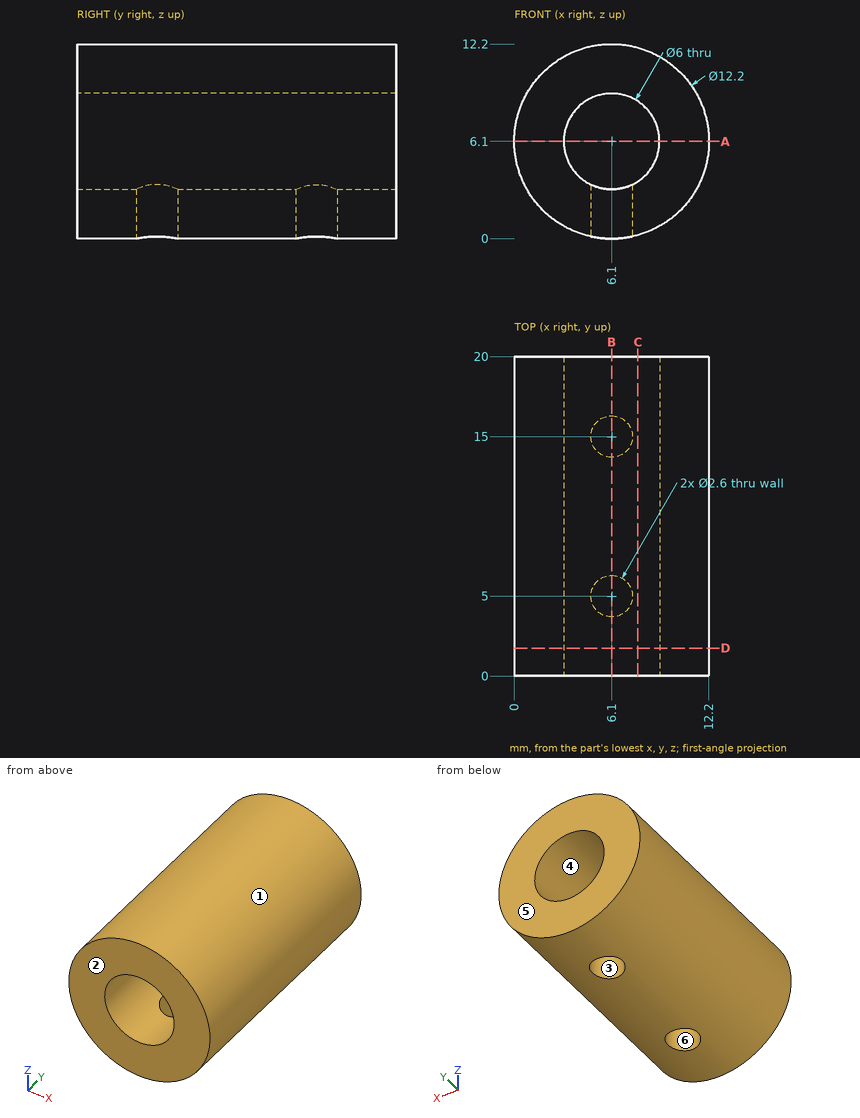
The drawing under review shows one solid part. Ordinate dimensions are in mm from its lowest x, y, z. A direction names the side the tool comes from. Coordinates: 2 decimals unless noted, no trailing zeros. Order: outer loops, then holes, each group sorted by start corner. A loop starts at its lowest first (then second) coordinate and runs counter-clockwise, first axis right, second up. Notation, with made-up numbers: (7.25, 47) -> (50.25, 47) arc R11 ccw to (50.25, 64) -> close; hole circle Ø11 at (67, 48.5). An arc over 180 degrees is marked (long way). Use CSV: the item, a comma, the result in double quotes. Start each with the question number.
Item 1: We need section C-C, the plane x = 7.75. Give the boundary of the cut face in (y, z), then the cut area to 3 significant figures.
Item 2: Insertion check: pin 1 (5 mm diameter, centred on x = 5.5, y = 3, fed in from -Z); pin 2 (5 mm diameter, centred on x = 10, y = 15.5, fed in from -Z); pin 3 (4 mm diameter, centred on y = 6, z = 1.5, fed in from +X); pin 4 (5 mm diameter, centred on x = 6.1, z = 6.1, fed in from +Y). Each pin has a flat end and moves straight along its axis. Give the tip position at first contact, or say it passes through.
Item 3: We need section A-A, the plane z = 6.1. Give the boundary of the cut face in (x, y), then the cut area to 3 significant figures.
Item 4: Draft analysis for pull direction X (two halves, no side actions). For the marked faces 1, 2, 3 and 4, state which applies: pulls with the +X half, pulls with the -X half, needs draft (parallel to the pull), parting line crosses it, or undercut.
Item 5: Wall thickness on probe 1 along Z at (x, y) = (6, 11.75); probe 2 along X at (y, z) = (15, 0.7): over which ranges is each line inside the solid? List them lowest first.
Item 6: For the marked faces 5 and 6, list the 3-axis set-ups (+Z, -Z, +X, -X, +Y, -Y) from which the entire face can be reached by the end or side of a thin tool; tool diameter is ignored.
Item 7: We need section D-D, the plane y = 1.75. Give the boundary of the cut face in (x, z).
Item 8: We need section B-B, the plane x = 6.1. Give the boundary of the cut face in (y, z).
Derived:
1,outline,"(0, 0.23) -> (20, 0.23) -> (20, 3.59) -> (0, 3.59) -> close; (0, 8.61) -> (20, 8.61) -> (20, 11.97) -> (0, 11.97) -> close"
1,area,"135 mm^2"
2,pin 1,"stops at z = 0"
2,pin 2,"stops at z = 0.16"
2,pin 3,"stops at x = 11.62"
2,pin 4,"passes through"
3,outline,"(0, 0) -> (3.1, 0) -> (3.1, 20) -> (0, 20) -> close; (9.1, 0) -> (12.2, 0) -> (12.2, 20) -> (9.1, 20) -> close"
3,area,"124 mm^2"
4,face 1,"parting line crosses it"
4,face 2,"needs draft"
4,face 3,"undercut"
4,face 4,"undercut"
5,probe 1,"z = 0 to 3.1, 9.1 to 12.2"
5,probe 2,"x = 3.26 to 4.8, 7.4 to 8.94"
6,face 5,"+Z, -Z, +X, -X, +Y"
6,face 6,"-Z"
7,outline,"circle Ø12.2 at (6.1, 6.1); hole circle Ø6 at (6.1, 6.1)"
8,outline,"(0, 0) -> (3.7, 0) -> (3.7, 3.1) -> (0, 3.1) -> close; (0, 9.1) -> (20, 9.1) -> (20, 12.2) -> (0, 12.2) -> close; (6.3, 0) -> (13.7, 0) -> (13.7, 3.1) -> (6.3, 3.1) -> close; (16.3, 0) -> (20, 0) -> (20, 3.1) -> (16.3, 3.1) -> close"
